CAD build for the part. Positions are in the model's coordinates, mm. Face numbers are marked on the shaded views. Give positions to 0.01 mm unless a question says otherwise; leave off trailing zeros. Order: outer loops, then holes, each group sorted by start corner. A loop starts at its lowest first (then second) coordinate and runs counter-clockwise, first axis right, second up.
Item 1: Wall check: L1, parallel to X at y = -3.65, z = 3.25; L2, parallel to X at y = -1.85, z = 2.25; L3, parallel to X at y = -2.9, z = 6.5. Give the ranges that are in metal, low to high.
Item 2: Band-saw the part on A-A on z = 4.5. Give the cut face in (x, y).
Item 3: Two-plate mould, pull along X, no slides. Class the marked faces 1, 2 and 3: released by +X, released by -X, zero draft, split by the parting line, or undercut.
Item 4: Flat gauge pin, fed straight in: P1, Ø3, axis at x = 13.65, y = -3.14, coming from the +Z side. Where does the tip first touch, or does it go through?
Item 5: Band-saw the part on D-D on z = 1. Give the cut face in (x, y).
Item 6: Band-saw the part on C-C on z = 7.25. Give the cut face in (x, y).
Item 7: Band-saw the part on B-B on y = -4.5. Give the cut face in (x, z).
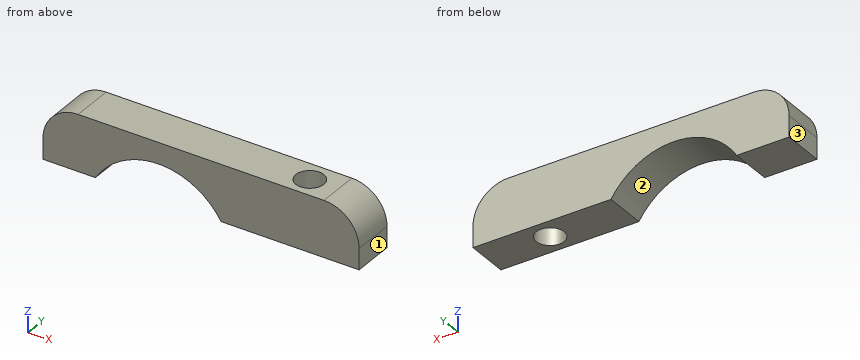
```python
from build123d import *

# Parameters (mm, degrees)
F0_W     = 45
F0_H     = 6
F0_R     = 2
F1_DEPTH = 8
F2_R     = 10.5
F3_DEPTH = 8
F4_R     = 5
F5_R     = 5


with BuildPart() as f1:
    # F0 (on Top) → F1 (new body)
    with BuildSketch(Plane.XY):
        with Locations((0.153442, -3.142335)):
            Rectangle(F0_W, F0_H)
        with Locations((13.653442, -3.142335)):
            Circle(F0_R, mode=Mode.SUBTRACT)
    extrude(amount=F1_DEPTH)

    # F2 (on Front) → F3 (cut)
    with BuildSketch(Plane.XZ):
        with Locations((-5.943397, -5.5)):
            Circle(F2_R)
    extrude(amount=F3_DEPTH, mode=Mode.SUBTRACT)

    # F4
    f4_edges = [f1.edges().sort_by_distance(p)[0] for p in [
        (-22.346558, -3.142335, 8),
    ]]
    fillet(f4_edges, radius=F4_R)

    # F5
    f5_edges = [f1.edges().sort_by_distance(p)[0] for p in [
        (22.653442, -3.142335, 8),
    ]]
    fillet(f5_edges, radius=F5_R)


solid = f1.part
```
The answers:
1. L1: x = -22.34 to -11.75, -0.14 to 11.72, 15.59 to 22.65
1. L2: x = -22.35 to -13.03, 1.14 to 12.13, 15.18 to 22.65
1. L3: x = -20.92 to 11.67, 15.64 to 21.22
2. outline: (-22.12, -6.14) - (-9.14, -6.14) - (-9.14, -0.14) - (-22.12, -0.14) - close; (-2.74, -6.14) - (22.42, -6.14) - (22.42, -0.14) - (-2.74, -0.14) - close; hole circle Ø4 at (13.65, -3.14)
3. face 1: released by +X
3. face 2: undercut
3. face 3: released by -X
4. P1: passes through
5. outline: (-22.35, -6.14) - (-14.19, -6.14) - (-14.19, -0.14) - (-22.35, -0.14) - close; (2.3, -6.14) - (22.65, -6.14) - (22.65, -0.14) - (2.3, -0.14) - close; hole circle Ø4 at (13.65, -3.14)
6. outline: (-19.98, -6.14) - (20.29, -6.14) - (20.29, -0.14) - (-19.98, -0.14) - close; hole circle Ø4 at (13.65, -3.14)
7. outline: (-22.35, 0) - (-14.89, 0) arc R10.5 cw to (3, 0) - (12.18, 0) - (12.18, 8) - (-17.35, 8) arc R5 ccw to (-22.35, 3) - close; (15.12, 0) - (22.65, 0) - (22.65, 3) arc R5 ccw to (17.65, 8) - (15.12, 8) - close
